```python
from build123d import *

# Parameters (mm, degrees)
BOSS_EXTRUDE1_DEPTH = 80
SKETCH3_R           = 1.5
CUT_EXTRUDE1_DEPTH  = 25
CUT_EXTRUDE2_REACH  = 27
SKETCH4_R           = 3


with BuildPart() as part:
    # Sketch2 → Boss-Extrude1 (new body)
    with BuildSketch(Plane.XY):
        Polygon((23, 25), (25, 25), (25, 0), (0, 0), (0, 25), (2, 25), (2, 2), (23, 2), align=None)
    extrude(amount=BOSS_EXTRUDE1_DEPTH)

    # Sketch3 → Cut-Extrude1 (cut)
    with BuildSketch(Plane(origin=(25, 0, 0), x_dir=(0, 0, -1), z_dir=(1, 0, 0))):
        with Locations((-65, 12.5)):
            Circle(SKETCH3_R)
    extrude(amount=-CUT_EXTRUDE1_DEPTH, mode=Mode.SUBTRACT)

    # Sketch4 → Cut-Extrude2 (cut, up to next)
    with BuildSketch(Plane.XZ, mode=Mode.PRIVATE) as cut_extrude2_sk1:
        with Locations((12.5, 60)):
            Circle(SKETCH4_R)
    cut_extrude2_tool1 = extrude(cut_extrude2_sk1.sketch, amount=-CUT_EXTRUDE2_REACH, mode=Mode.PRIVATE) & part.part
    add(cut_extrude2_tool1.solids().sort_by_distance((12.5, 0, 60))[0], mode=Mode.SUBTRACT)
    # Sketch4 → Cut-Extrude2 (cut, up to next)
    with BuildSketch(Plane.XZ, mode=Mode.PRIVATE) as cut_extrude2_sk2:
        with Locations((12.5, 20)):
            Circle(SKETCH4_R)
    cut_extrude2_tool2 = extrude(cut_extrude2_sk2.sketch, amount=-CUT_EXTRUDE2_REACH, mode=Mode.PRIVATE) & part.part
    add(cut_extrude2_tool2.solids().sort_by_distance((12.5, 0, 20))[0], mode=Mode.SUBTRACT)


solid = part.part
```
Check sheet for the modelled part. Datum: model origin and axes. Units: mm. A direction names the side the tool comes from. Coordinates: 2 decimals unless noted, no trailing zeros. Order: outer loops, then holes, each group sorted by start corner. A loop starts at its lowest first (then second) coordinate and runs counter-clockwise, first axis right, second up. Notation, with made-up numbers: (-6.5, 54.25) -> (42.5, 54.25) arc R13 cw to (42.5, 73.25) -> close; hole circle Ø3 at (63, -32.75). An arc over 180 degrees is marked (long way). Write item = value, one per line. Start each with the question number.
1) Cross-section at B-B (z = 65). Enter the section's corners in (x, y), then the cut area to 3 significant figures.
2) Mould release check, pull along Z, two halves, no side actions. Record for faces 1 (the flat face through (1, 25, 39)), 2 (the flat face through (13, 1, 0)), 3 (the cylindrical face through (10.1, 1, 18.2)): +Z half, -Z half, draft (parallel to the pull), parting line (faces both ways), or undercut.
3) Go/stop test with flat-tipped pins: P1, Ø10.5, axis at x = 8, z = 35, coming from the +Y side; P2, Ø1, axis at x = 19, z = 69.5, coming from the -Y side. Record where each tip stops, or that it passes through.
4) Cross-section at A-A (y = 7). Enter the section's corners in (x, z).
5) Cross-section at D-D (z = 18). Enter the section's corners in (x, y), then the cut area to 3 significant figures.
6) Material ranges on L1, parallel to Z at x = 12.5, y = 1.45; L2, parallel to X at y = 4.5, z = 72; L3, parallel to Y at x = 23.75, z = 65, recorded low to high.
7) Access from +Z, -Z, +X, -X, +Y, -Y to the whole of each face (thin tool, end or side, straight path). Record for faces 4 (the flat face through (12, 2, 39)), 5 (the flat face through (25, 13, 39)).
8) Cross-section at C-C (x = 11.25). Enter the section's corners in (y, z).
Ans:
q1.outline = (0, 0) -> (25, 0) -> (25, 11) -> (23, 11) -> (23, 2) -> (2, 2) -> (2, 11) -> (0, 11) -> close; (0, 14) -> (2, 14) -> (2, 25) -> (0, 25) -> close; (23, 14) -> (25, 14) -> (25, 25) -> (23, 25) -> close
q1.area = 130 mm²
q2.face_1 = draft
q2.face_2 = -Z half
q2.face_3 = undercut
q3.P1 = 2
q3.P2 = 0
q4.outline = (0, 0) -> (2, 0) -> (2, 80) -> (0, 80) -> close; (23, 0) -> (25, 0) -> (25, 80) -> (23, 80) -> close
q5.outline = (0, 0) -> (10.26, 0) -> (10.26, 2) -> (2, 2) -> (2, 25) -> (0, 25) -> close; (14.74, 0) -> (25, 0) -> (25, 25) -> (23, 25) -> (23, 2) -> (14.74, 2) -> close
q5.area = 133 mm²
q6.L1 = 0 to 17, 23 to 57, 63 to 80
q6.L2 = 0 to 2, 23 to 25
q6.L3 = 0 to 11, 14 to 25
q7.face_4 = +Z, -Z, +Y
q7.face_5 = +Z, -Z, +X, +Y, -Y
q8.outline = (0, 0) -> (2, 0) -> (2, 17.27) -> (0, 17.27) -> close; (0, 22.73) -> (2, 22.73) -> (2, 57.27) -> (0, 57.27) -> close; (0, 62.73) -> (2, 62.73) -> (2, 80) -> (0, 80) -> close
